Geometry check sheet. Reference: drawing and pictorial views, mm from the part's lowest x, y, z. A direction names the side the tool comes from. Round coordinates to 2 decimals unless told otherwise and drop trailing zeros. Order: outer loops, then holes, each group sorted by start corner. A loop starts at its lowest first (then second) coordinate and runs counter-clockwise, first axis right, second up.
Q1. Mould release check, pull along Z, two halves, no side actions. Record for the marked faces 1, 2 and 3: +Z half, -Z half, draft (parallel to the pull), parting line (faces both ways), or undercut.
Q2. Set-up check for the marked faces 4 and 5: record each of +Z, -Z, +X, -X, +Y, -Y from which the full face is reachable in a straight line by a thin tool's end or side.
Q3. Cross-section at A-A on x = 10. Record the cut outline in (y, z).
Q4. Cross-section at C-C on z = 10. Record the cut outline in (x, y).
Q5. Cross-section at D-D on y = 2.55. Record the cut outline in (x, z), then the cut area to 3 significant figures.
Q6. Depth check by flat-ended pin: P1, Ø2.5, axis at x = 8.07, z = 6.91, coming from the +Y side; P2, Ø2, axis at y = 1, z = 17, coming from the +X side; P3, Ø1.5, axis at x = 8, y = 2, coming from the +Z side. Enter the tip coordinate at first touch or a pass-through.
Q7. Scan lines: probe 1 along X at (y, z) = (1.2, 13.25); probe 2 along Y at (x, z) = (11.75, 14); probe 3 along Z at (x, y) = (11.5, 4.4). Record each from-to range of solid material in increasing order.
Q8. Cross-section at B-B on y = 4.6. Record the cut outline in (x, z).
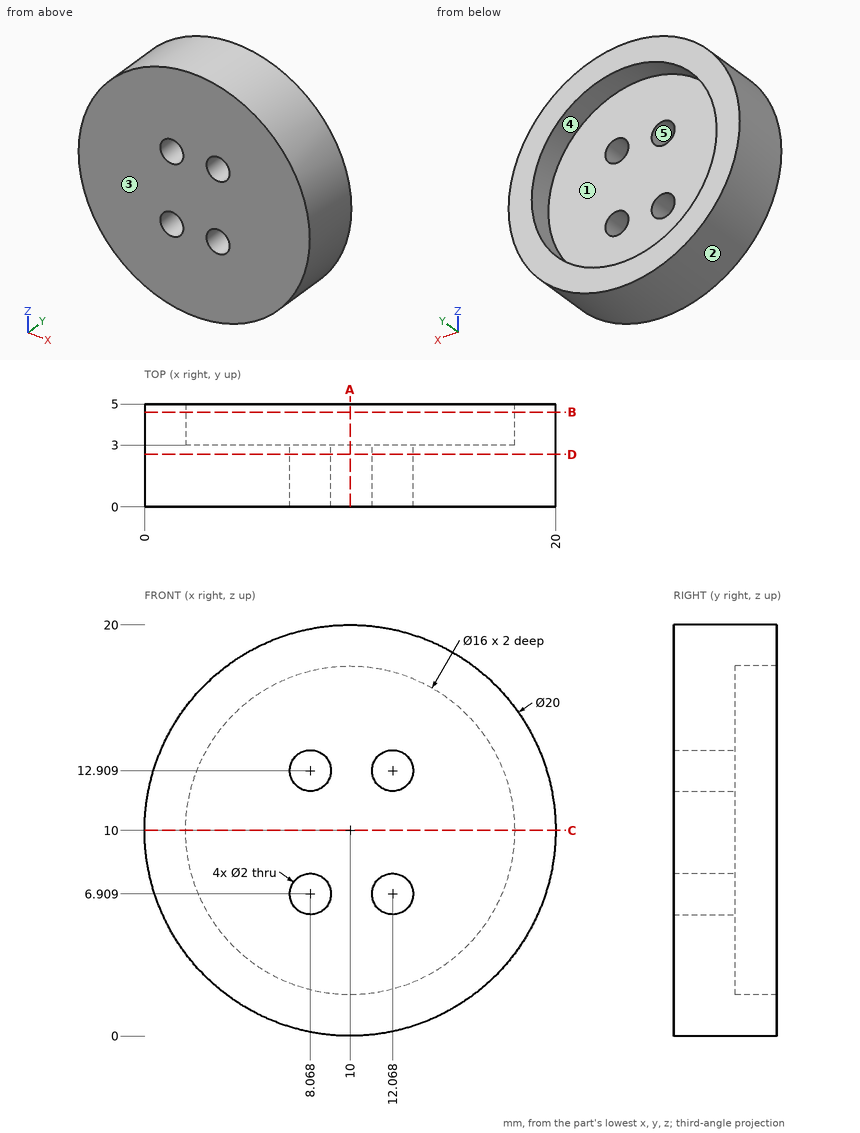
Results found:
1. face 1: undercut
1. face 2: parting line
1. face 3: draft
2. face 4: +Y
2. face 5: +Y, -Y
3. outline: (0, 0) - (5, 0) - (5, 2) - (3, 2) - (3, 18) - (5, 18) - (5, 20) - (0, 20) - close
4. outline: (0, 0) - (20, 0) - (20, 5) - (18, 5) - (18, 3) - (2, 3) - (2, 5) - (0, 5) - close
5. outline: circle Ø20 at (10, 10); hole circle Ø2 at (8.07, 6.91); hole circle Ø2 at (8.07, 12.91); hole circle Ø2 at (12.07, 6.91); hole circle Ø2 at (12.07, 12.91)
5. area: 302 mm2
6. P1: stops at y = 3
6. P2: stops at x = 18
6. P3: stops at z = 19.92
7. probe 1: x = 0.54 to 7.13, 9.01 to 11.13, 13.01 to 19.46
7. probe 2: y = 0 to 3
7. probe 3: z = 0.11 to 2.14, 17.86 to 19.89
8. outline: circle Ø20 at (10, 10); hole circle Ø16 at (10, 10)
